```python
from build123d import *

# Parameters (mm, degrees)
SKETCH1_W               = 8.9916
SKETCH1_H               = 3.302
BOSS_EXTRUDE1_DEPTH     = 3.5052
SKETCH2_W               = 1.4986
SKETCH2_H               = 1.4986
BOSS_EXTRUDE2_DEPTH     = 2.0066
FILLET1_R               = 0.5
SKETCH3_W               = 0.6096
SKETCH3_H               = 0.3048
BOSS_EXTRUDE3_DEPTH     = 2.9972
LPATTERN1_COUNT         = 3
LPATTERN1_PITCH         = 2.4892
MIRROR6_COPY_1_SKETCH_W = 0.6096
MIRROR6_COPY_1_SKETCH_H = 0.3048
MIRROR6_COPY_1_DEPTH    = 2.9972
MIRROR6_COPY_2_SKETCH_W = 0.6096
MIRROR6_COPY_2_SKETCH_H = 0.3048
MIRROR6_COPY_2_DEPTH    = 2.9972


with BuildPart() as part:
    # Sketch1 → Boss-Extrude1 (new body)
    with BuildSketch(Plane(origin=(0, 0, 0), x_dir=(1, 0, 0), z_dir=(0, 1, 0))):
        Rectangle(SKETCH1_W, SKETCH1_H)
    extrude(amount=BOSS_EXTRUDE1_DEPTH)

    # Sketch2 → Boss-Extrude2 (add)
    with BuildSketch(Plane.XY.offset(1.651)):
        with Locations((-1.0033, 2.4892)):
            Rectangle(SKETCH2_W, SKETCH2_H)
    extrude(amount=BOSS_EXTRUDE2_DEPTH)

    # Fillet1
    fillet1_edges = [part.edges().sort_by_distance(p)[0] for p in [
        (4.4958, 3.5052, 0),
        (-4.4958, 3.5052, 0),
    ]]
    fillet(fillet1_edges, radius=FILLET1_R)

    # Sketch3 → Boss-Extrude3 (add)
    with BuildSketch(Plane.XZ):
        with Locations((2.4892, 1.4986)):
            Rectangle(SKETCH3_W, SKETCH3_H)
    boss_extrude3 = extrude(amount=BOSS_EXTRUDE3_DEPTH)

    # LPattern1: Boss-Extrude3 ×3
    with Locations(*[(-i * LPATTERN1_PITCH, 0, 0) for i in range(1, LPATTERN1_COUNT)]):
        add(boss_extrude3)

    # Mirror6: Boss-Extrude3 across plane
    add(boss_extrude3.mirror(Plane.XY))

    # Mirror6 copy 1 sketch → Mirror6 copy 1 (add)
    with BuildSketch(Plane(origin=(-2.4892, 0, 0), x_dir=(1, 0, 0), z_dir=(0, -1, 0))):
        with Locations((2.4892, -1.4986)):
            Rectangle(MIRROR6_COPY_1_SKETCH_W, MIRROR6_COPY_1_SKETCH_H)
    extrude(amount=MIRROR6_COPY_1_DEPTH)

    # Mirror6 copy 2 sketch → Mirror6 copy 2 (add)
    with BuildSketch(Plane(origin=(-4.9784, 0, 0), x_dir=(1, 0, 0), z_dir=(0, -1, 0))):
        with Locations((2.4892, -1.4986)):
            Rectangle(MIRROR6_COPY_2_SKETCH_W, MIRROR6_COPY_2_SKETCH_H)
    extrude(amount=MIRROR6_COPY_2_DEPTH)


solid = part.part
```
For this review, take the finished solid that the model builds, in its own axes (mm). A direction names the side the tool comes from. Round coordinates to 2 decimals unless told otherwise and drop trailing zeros. Write each loop counter-clockwise with the first axis right and the second up, starting at its lowest first coordinate (ties: lowest second). Pieces come first, ordered by that corner, then holes. Notation, with made-up numbers: (-2, 32.5) - (31, 32.5) arc R20 cw to (31, 71.5) - close; hole circle Ø2 at (-32.75, 52). An arc over 180 degrees is marked (long way). Answer as a JSON object with one key per item and string values.
1. We need section C-C on y = 2.5. Give the boundary of the cut face in (x, z).
Response values:
{"outline": "(-4.5, -1.65) - (4.5, -1.65) - (4.5, 1.65) - (-0.25, 1.65) - (-0.25, 3.66) - (-1.75, 3.66) - (-1.75, 1.65) - (-4.5, 1.65) - close"}
2. Tool access review of faces 1 (the face through (-1.753, 2, 3)), 2 (the face through (-0.254, 2, 3)), 3 (the face through (-4.496, 1, 0)), 4 (the face through (-1, 3.238, 3)), 5 (the face through (-1, 1.74, 3)): name each direction out of +Z, -Z, +X, -X, +Y, -Y from which nothing blocks a thin tool from reaching the whole face with its end or side.
Response values:
{"face 1": "+Z, -X, +Y, -Y", "face 2": "+Z, +X, +Y, -Y", "face 3": "+Z, -Z, -X, +Y, -Y", "face 4": "+Z, +X, -X, +Y", "face 5": "+Z, +X, -X, -Y"}
3. To check wall thickness, follow line 1 along X through (y, z) = (-2.5, 1.4); line 2 along Y through (x, z) = (-1, -0.8); line 3 along Z through (x, y) = (-2, 2). State the ranges of each line that lie inside material, in increasing order.
Response values:
{"line 1": "x = -2.79 to -2.18, -0.3 to 0.3, 2.18 to 2.79", "line 2": "y = 0 to 3.51", "line 3": "z = -1.65 to 1.65"}
4. We need section B-B on x = -0.75. Give the boundary of the cut face in (y, z).
Response values:
{"outline": "(0, -1.65) - (3.51, -1.65) - (3.51, 1.65) - (3.24, 1.65) - (3.24, 3.66) - (1.74, 3.66) - (1.74, 1.65) - (0, 1.65) - close"}
5. We need section A-A on y = -1.5. Give the boundary of the cut face in (x, z).
Response values:
{"outline": "(-2.79, -1.65) - (-2.18, -1.65) - (-2.18, -1.35) - (-2.79, -1.35) - close; (-2.79, 1.35) - (-2.18, 1.35) - (-2.18, 1.65) - (-2.79, 1.65) - close; (-0.3, -1.65) - (0.3, -1.65) - (0.3, -1.35) - (-0.3, -1.35) - close; (-0.3, 1.35) - (0.3, 1.35) - (0.3, 1.65) - (-0.3, 1.65) - close; (2.18, -1.65) - (2.79, -1.65) - (2.79, -1.35) - (2.18, -1.35) - close; (2.18, 1.35) - (2.79, 1.35) - (2.79, 1.65) - (2.18, 1.65) - close"}
6. For pin 1 Ø1 at (y, z) = (-2, 0.5) entering from -X; pin 2 Ø0.5 at (x, y) = (0, -1) entering from +Z; pin 3 Ø2 at (x, z) = (-1.5, 0.5) entering from -Y; pin 4 Ø0.7 at (y, z) = (3, 3) entering from +X, all flat-tipped, find the tip position at first contact; note any pin that passes through.
Response values:
{"pin 1": "passes through", "pin 2": "stops at z = 1.65", "pin 3": "stops at y = 0", "pin 4": "stops at x = -0.25"}
7. We need section D-D on z = 1.55. Give the boundary of the cut face in (x, y), then the cut area to 3 significant figures.
Response values:
{"outline": "(-4.5, 0) - (-2.79, 0) - (-2.79, -3) - (-2.18, -3) - (-2.18, 0) - (-0.3, 0) - (-0.3, -3) - (0.3, -3) - (0.3, 0) - (2.18, 0) - (2.18, -3) - (2.79, -3) - (2.79, 0) - (4.5, 0) - (4.5, 3.01) arc R0.5 ccw to (4, 3.51) - (-4, 3.51) arc R0.5 ccw to (-4.5, 3.01) - close", "area": "36.9 mm2"}
